```python
from build123d import *

# Parameters (mm, degrees)
SKETCH_1_W                = 20
SKETCH_1_H                = 20
EXTRUDE_1_DEPTH           = 40
SKETCH_2_W                = 10
SKETCH_2_H                = 15
CUT_EXTRUDE_1_DEPTH       = 7.071067812
PATTERN_CIRCULAR_1_COUNT  = 4
SKETCH_5_R                = 3.5
CUT_EXTRUDE_2_DEPTH       = 25
CUT_EXTRUDE_3_DEPTH       = 5
SKETCH_9_W                = 5.878932188
SKETCH_9_H                = 5.878932188
CUT_EXTRUDE_5_DEPTH       = 5
SKETCH_11_W               = 10
SKETCH_11_H               = 30
EXTRUDE_2_DEPTH           = 10
CUT_EXTRUDE_6_DEPTH       = 30
SKETCH_13_R               = 1.25
CUT_EXTRUDE_7_DEPTH       = 10
PATTERN_CIRCULAR_2_COUNT  = 4
SKETCH_16_W               = 20
SKETCH_16_H               = 10
CUT_EXTRUDE_11_DEPTH      = 40
SKETCH_17_W               = 20
SKETCH_17_H               = 20
SKETCH_17_W_2             = 5.857864376
SKETCH_17_H_2             = 5.857864376
CUT_EXTRUDE_12_DEPTH      = 5
CUT_EXTRUDE_13_DEPTH      = 54.851648071
CUT_EXTRUDE_13_DEPTH_BACK = 10
SKETCH_19_W               = 81.536041923
SKETCH_19_H               = 68.786769913
CUT_EXTRUDE_16_DEPTH      = 400
SKETCH_20_W               = 73.081310303
SKETCH_20_H               = 44.358386444
CUT_EXTRUDE_18_DEPTH      = 400


with BuildPart() as part:
    # 스케치1 → 보스-돌출1 (new body)
    with BuildSketch(Plane.XY):
        Rectangle(SKETCH_1_W, SKETCH_1_H)
    extrude(amount=EXTRUDE_1_DEPTH)

    # 스케치2 → 컷-돌출1 (cut)
    with BuildSketch(Plane(origin=(10, 0, 0), x_dir=(0, 0, -1), z_dir=(1, 0, 0))):
        with Locations((-10, 0)):
            Rectangle(SKETCH_2_W, SKETCH_2_H)
    cut_extrude_1 = extrude(amount=-CUT_EXTRUDE_1_DEPTH, mode=Mode.SUBTRACT)

    # 원형 패턴1: 컷-돌출1 ×4 about axis
    pattern_circular_1_axis = Axis((0, 0, 0), (0, 0, 1))
    for i in range(1, PATTERN_CIRCULAR_1_COUNT):
        add(cut_extrude_1.rotate(pattern_circular_1_axis, i * 360 / PATTERN_CIRCULAR_1_COUNT), mode=Mode.SUBTRACT)

    # 스케치5 → 컷-돌출2 (cut)
    with BuildSketch(Plane.XY.offset(40)):
        with Locations((-5.5, 5.5)):
            Circle(SKETCH_5_R)
        with Locations((5.5, 5.5)):
            Circle(SKETCH_5_R)
        with Locations(Location((-5.5, -5.5, 0), (0, 0, 235.150095421))):
            Circle(SKETCH_5_R)
        with Locations(Location((5.5, -5.5, 0), (0, 0, 304.849904579))):
            Circle(SKETCH_5_R)
    extrude(amount=-CUT_EXTRUDE_2_DEPTH, mode=Mode.SUBTRACT)

    # 스케치6 → 컷-돌출3 (cut)
    with BuildSketch(Plane(origin=(0, 0, 0), x_dir=(-1, 0, 0), z_dir=(0, 0, -1))):
        Polygon((-14.808802863, -2.95), (-14.808802863, 2.95), (-2.95, 2.95), (-2.95, 12.360254216), (2.95, 12.360254216), (2.95, 2.95), (13.852115441, 2.95), (13.852115441, -2.95), (2.95, -2.95), (2.95, -13.975695818), (-2.95, -13.975695818), (-2.95, -2.95), align=None)
    extrude(amount=-CUT_EXTRUDE_3_DEPTH, mode=Mode.SUBTRACT)

    # 스케치9 → 컷-돌출5 (cut)
    with BuildSketch(Plane(origin=(0, 0, 5), x_dir=(-1, 0, 0), z_dir=(0, 0, -1))):
        with Locations((0.010533906, -0.010533906)):
            Rectangle(SKETCH_9_W, SKETCH_9_H)
    extrude(amount=-CUT_EXTRUDE_5_DEPTH, mode=Mode.SUBTRACT)

    # 스케치11 → 보스-돌출2 (add)
    with BuildSketch(Plane(origin=(10, 0, 0), x_dir=(0, 0, -1), z_dir=(1, 0, 0))):
        with Locations((-20, 0)):
            Rectangle(SKETCH_11_W, SKETCH_11_H)
    extrude_2 = extrude(amount=EXTRUDE_2_DEPTH)

    # 스케치12 → 컷-돌출6 (cut)
    with BuildSketch(Plane(origin=(0, 15, 0), x_dir=(1, 0, 0), z_dir=(0, 1, 0))):
        Polygon((20, -15), (10, -25), (20, -25), align=None)
    cut_extrude_6 = extrude(amount=-CUT_EXTRUDE_6_DEPTH, mode=Mode.SUBTRACT)

    # 스케치13 → 컷-돌출7 (cut)
    with BuildSketch(Plane(origin=(0, 0, 15), x_dir=(-1, 0, 0), z_dir=(0, 0, -1))):
        with Locations(Location((-15, -5, 0), (0, 0, 90))):
            Circle(SKETCH_13_R)
        with Locations(Location((-15, 5, 0), (0, 0, 90))):
            Circle(SKETCH_13_R)
    cut_extrude_7 = extrude(amount=-CUT_EXTRUDE_7_DEPTH, mode=Mode.SUBTRACT)

    # 원형 패턴2: 보스-돌출2, 컷-돌출6, 컷-돌출7 ×4 about axis
    pattern_circular_2_axis = Axis((0, 0, 0), (0, 0, 1))
    add([extrude_2.rotate(pattern_circular_2_axis, i * 360 / PATTERN_CIRCULAR_2_COUNT) for i in range(1, PATTERN_CIRCULAR_2_COUNT)])
    add([cut_extrude_6.rotate(pattern_circular_2_axis, i * 360 / PATTERN_CIRCULAR_2_COUNT) for i in range(1, PATTERN_CIRCULAR_2_COUNT)], mode=Mode.SUBTRACT)
    add([cut_extrude_7.rotate(pattern_circular_2_axis, i * 360 / PATTERN_CIRCULAR_2_COUNT) for i in range(1, PATTERN_CIRCULAR_2_COUNT)], mode=Mode.SUBTRACT)

    # 스케치16 → 컷-돌출11 (cut)
    with BuildSketch(Plane.XZ.offset(10)):
        with Locations((0, 5)):
            Rectangle(SKETCH_16_W, SKETCH_16_H)
    extrude(amount=-CUT_EXTRUDE_11_DEPTH, mode=Mode.SUBTRACT)

    # 스케치17 → 컷-돌출12 (cut)
    with BuildSketch(Plane(origin=(0, 0, 10), x_dir=(-1, 0, 0), z_dir=(0, 0, -1))):
        Rectangle(SKETCH_17_W, SKETCH_17_H)
        Rectangle(SKETCH_17_W_2, SKETCH_17_H_2, mode=Mode.SUBTRACT)
    extrude(amount=-CUT_EXTRUDE_12_DEPTH, mode=Mode.SUBTRACT)

    # 스케치18 → 컷-돌출13 (cut, two sides: drawn at the far end of the back side and taken through both)
    with BuildSketch(Plane.XZ.offset(-10).offset(-CUT_EXTRUDE_13_DEPTH_BACK)):
        Polygon((10, 25), (15, 25), (15, 20), align=None)
    extrude(amount=CUT_EXTRUDE_13_DEPTH + CUT_EXTRUDE_13_DEPTH_BACK, mode=Mode.SUBTRACT)

    # 스케치19 → 컷-돌출16 (cut)
    with BuildSketch(Plane(origin=(0, 0, 0), x_dir=(1, 0, 0), z_dir=(0, 1, 0))):
        with Locations((9.636077682, -26.334226141)):
            Rectangle(SKETCH_19_W, SKETCH_19_H)
    extrude(amount=-CUT_EXTRUDE_16_DEPTH, mode=Mode.SUBTRACT)

    # 스케치20 → 컷-돌출18 (cut)
    with BuildSketch(Plane(origin=(0, 0, 0), x_dir=(0, 0, -1), z_dir=(1, 0, 0))):
        with Locations((-16.834813983, 6.467543638)):
            Rectangle(SKETCH_20_W, SKETCH_20_H)
    extrude(amount=-CUT_EXTRUDE_18_DEPTH, mode=Mode.SUBTRACT)


solid = part.part
```
Check sheet for the modelled part. Datum: model origin and axes. Units: mm. A direction names the side the tool comes from. Coordinates: 2 decimals unless noted, no trailing zeros. Write each loop counter-clockwise with the first axis right and the second up, starting at its lowest first coordinate (ties: lowest second). Pieces come first, ordered by that corner, then holes. Notation, with made-up numbers: (39, -12.5) - (51, -12.5) arc R19 ccw to (51, 1.5) - close; hole circle Ø11 at (-38.75, 2). An arc over 180 degrees is marked (long way). One line per question, with ' | ' between items.
Item 1: Mould release check, pull along Y, two halves, no side actions. Record for faces 5 (the face through (5, 0, 28)), 6 (the face through (13.891, 5.577, 17.398)), 7 (the face through (2.7, 2.8, 40)), 8 (the face through (7.115, 2.395, 27.675)): pulls with the +Y half, pulls with the -Y half, needs draft (parallel to the pull), parting line crosses it, or undercut.
Determined:
face 5: pulls with the -Y half | face 6: undercut | face 7: needs draft | face 8: undercut
Item 2: Thickness scan on line 1 (X direction, y = 4, z = 15.5); line 2 (Z direction, x = 9.75, y = 2.75); line 3 (Y direction, x = 16.75, z = 16.25). Record the ranges inside material, lowest first. Write a range as [from, to].
Determined:
line 1: x = [0, 2.34], [8.66, 14.25], [15.75, 19.5] | line 2: z = [15, 40] | line 3: y = [0, 15]
Item 3: Sectioned sample at D-D on z = 31.25. Record the boundary of the cut face in (x, y), plus the area to 3 significant figures.
Determined:
outline: (0, 0) - (10, 0) - (10, 10) - (0, 10) - close; hole circle Ø7 at (5.5, 5.5) | area: 61.5 mm2
Item 4: Gauge pin test, flat ends, axial feed: P1, Ø1.5, axis at x = 2, z = 12.5, coming from the +Y side; P2, Ø8, axis at x = 2.5, z = 17, coming from the -Y side; P3, Ø5, axis at x = 7, z = 33, coming from the +Y side; P4, Ø5, axis at x = 11, y = 16, coming from the +Z side. Record the tip position at first contact, or that the pin passes through.
Determined:
P1: stops at y = 2.93 | P2: stops at y = 0 | P3: stops at y = 10 | P4: stops at z = 21.5
Item 5: Access from +Z, -Z, +X, -X, +Y, -Y to the whole of each face (thin tool, end or side, straight path). Record for faces 1 (the face through (10, 5, 32)), 2 (the face through (5, 10, 32)), 3 (the face through (15, 16, 16)), 4 (the face through (2.929, 1, 13)).
Determined:
face 1: +Z, +X, +Y, -Y | face 2: +Z, +X, -X, +Y | face 3: +Z, -Z, +X, +Y | face 4: -Z, +X, +Y, -Y
Item 6: Sectioned sample at A-A on z = 17. Record the boundary of the cut face in (x, y).
Determined:
outline: (0, 0) - (18, 0) - (18, 15) - (15, 15) - (15, 18) - (0, 18) - close; hole circle Ø7 at (5.5, 5.5); hole circle Ø2.5 at (5, 15); hole circle Ø2.5 at (15, 5)
Item 7: Sectioned sample at C-C on y = 5.5. Record the boundary of the cut face in (x, z), plus the area to 3 significant figures.
Determined:
outline: (0, 15) - (2, 15) - (2, 40) - (0, 40) - close; (9, 15) - (13.85, 15) - (13.85, 21.15) - (10, 25) - (10, 40) - (9, 40) - close; (16.15, 15) - (20, 15) - (16.15, 18.85) - close | area: 114 mm2
Item 8: Sectioned sample at B-B on x = 5. Record the boundary of the cut face in (y, z).
Determined:
outline: (0, 15) - (2.04, 15) - (2.04, 40) - (0, 40) - close; (8.96, 15) - (13.75, 15) - (13.75, 21.25) - (10, 25) - (10, 40) - (8.96, 40) - close; (16.25, 15) - (20, 15) - (16.25, 18.75) - close
